Study the drawing (mm; zero at the part's minimum x, y, z) and answer. A direction names the side the tool comes from. Give positions to 0.01 mm unless a question says otherwise; leave off trailing zeros. Loops run counter-clockwise (first coordinate to the right, second up) from the corner with the lowest first, then second, coordinate; pieces in that order, holes last. Notation, with made-up numbers: M 34,73.5 L 52,73.5 A16 ccw 52,79.5 Z; hole C 40,2.5 d11. An arc over 180 degrees is marked long. Return JSON: item names as keys, results as strings.
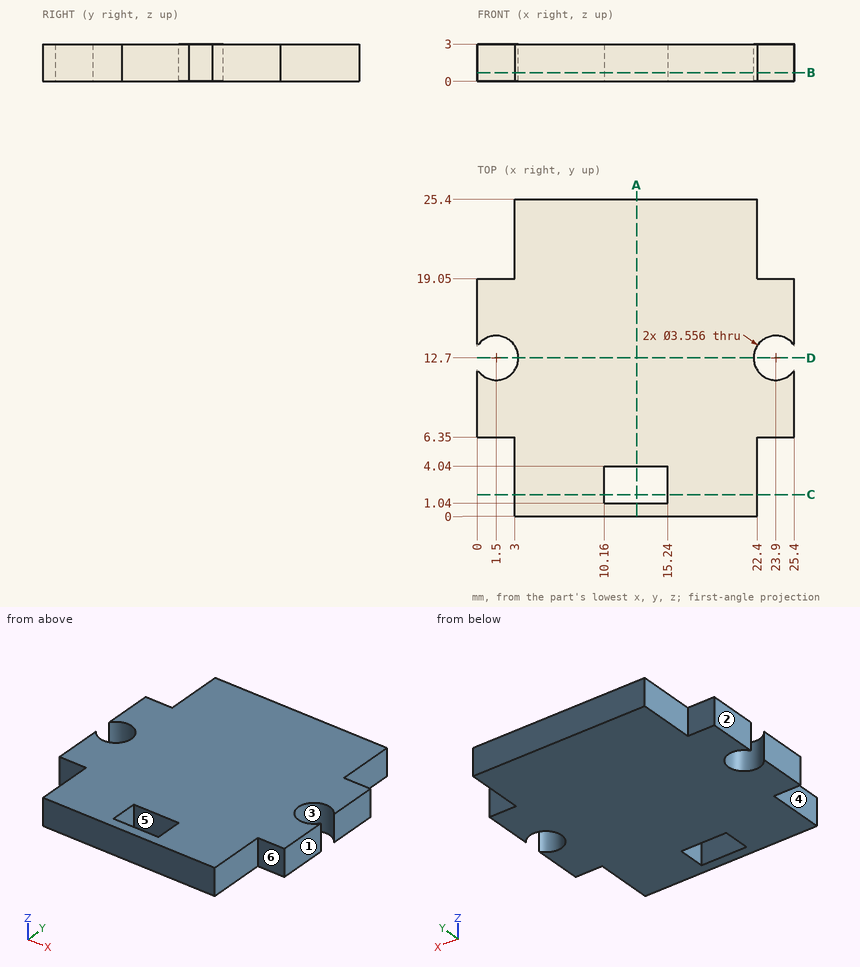
(1) The part is cut by section D-D (y = 12.7). Determine the outline of the cut face in (x, z).
Values follow:
{"outline": "M 3.28,0 L 22.12,0 L 22.12,3 L 3.28,3 Z"}
(2) The part is cut by section B-B (z = 0.7). Determine the outline of the cut face in (x, y), and give its area (3 significant figures).
Values follow:
{"outline": "M 0,6.35 L 3,6.35 L 3,0 L 22.4,0 L 22.4,6.35 L 25.4,6.35 L 25.4,11.75 A1.78 cw long 25.4,13.65 L 25.4,19.05 L 22.4,19.05 L 22.4,25.4 L 3,25.4 L 3,19.05 L 0,19.05 L 0,13.65 A1.78 cw long 0,11.75 Z; hole M 10.16,1.04 L 15.24,1.04 L 15.24,4.04 L 10.16,4.04 Z", "area": "535 mm²"}
(3) Determine the mould class of the marked faces 1, 2 and 3 for opening direction X: released by +X, released by -X, zero draft, split by the parting line, or undercut.
Values follow:
{"face 1": "released by +X", "face 2": "released by -X", "face 3": "undercut"}
(4) Given pin 1 (1.5 mm diameter, centred on x = 23.5, z = 2, fed in from +Y); pin 2 (1.5 mm diameter, centred on y = 2.5, z = 2, fed in from -X); pin 3 (1.5 mm diameter, centred on y = 2, z = 1, fed in from +X), each flat-ended and moving along its own axis, determine where each tip first touches the part or whether it passes through.
Values follow:
{"pin 1": "y = 19.05", "pin 2": "x = 3", "pin 3": "x = 22.4"}
(5) Straight lines are drawn through the part: line 1 along Y through (x, z) = (23.9, 1.1); line 2 along Y through (x, z) = (12.75, 1.4); line 3 along X through (y, z) = (2.75, 0.75). For each, find the intervals that lie inside material, in ascending order.
Values follow:
{"line 1": "6.35 to 10.92, 14.48 to 19.05", "line 2": "0 to 1.04, 4.04 to 25.4", "line 3": "3 to 10.16, 15.24 to 22.4"}
(6) The part is cut by section A-A (x = 12.75). Determine the outline of the cut face in (y, z).
Values follow:
{"outline": "M 0,0 L 1.04,0 L 1.04,3 L 0,3 Z; M 4.04,0 L 25.4,0 L 25.4,3 L 4.04,3 Z"}
(7) The part is cut by section C-C (y = 1.75). Determine the outline of the cut face in (x, z), and give its area (3 significant figures).
Values follow:
{"outline": "M 3,0 L 10.16,0 L 10.16,3 L 3,3 Z; M 15.24,0 L 22.4,0 L 22.4,3 L 15.24,3 Z", "area": "43.0 mm²"}
(8) A tool of negligible diameter and unlimited length cuts with its end or side. For the marked faces 4, 5 and 6, from which of +Z, -Z, +X, -X, +Y, -Y can it reach the whole face along a straight path? Write none if from no direction.
Values follow:
{"face 4": "+Z, -Z, -X, -Y", "face 5": "+Z, -Z", "face 6": "+Z, -Z, +X, -Y"}
